Geometry check sheet. Reference: drawing and pictorial views, mm from the part's lowest x, y, z. Give positions to 0.01 mm unless a question says otherwise; leave off trailing zeros. Loops run counter-clockwise (first coordinate to the right, second up) from the corner with the lowest first, then second, coordinate; pieces in that order, holes last. Notation, with made-up numbers: (-14.75, 3.5) - (-5.75, 3.5) arc R28 ccw to (-5.75, 35.5) - close; hole circle Ø4 at (22, -36). An arc over 180 degrees is marked (long way). One line per question, with ' | ' between items. Start each with the question number.
1. Thickness scan on line 1 along Z through (x, y) = (182.5, 1.5); line 2 along X through (y, z) = (9, 563.5). Record the ranges inside material, lowest first. Write a range as from..to.
2. Section check A-A, the plane z = 652. Enter the section's corners in (x, y).
3. Section check C-C, the plane x = 187.5. Enter the section's corners in (y, z).
4. Section check B-B, the plane y = 3.5. Enter the section's corners in (x, z), then the cut area to 3 significant figures.
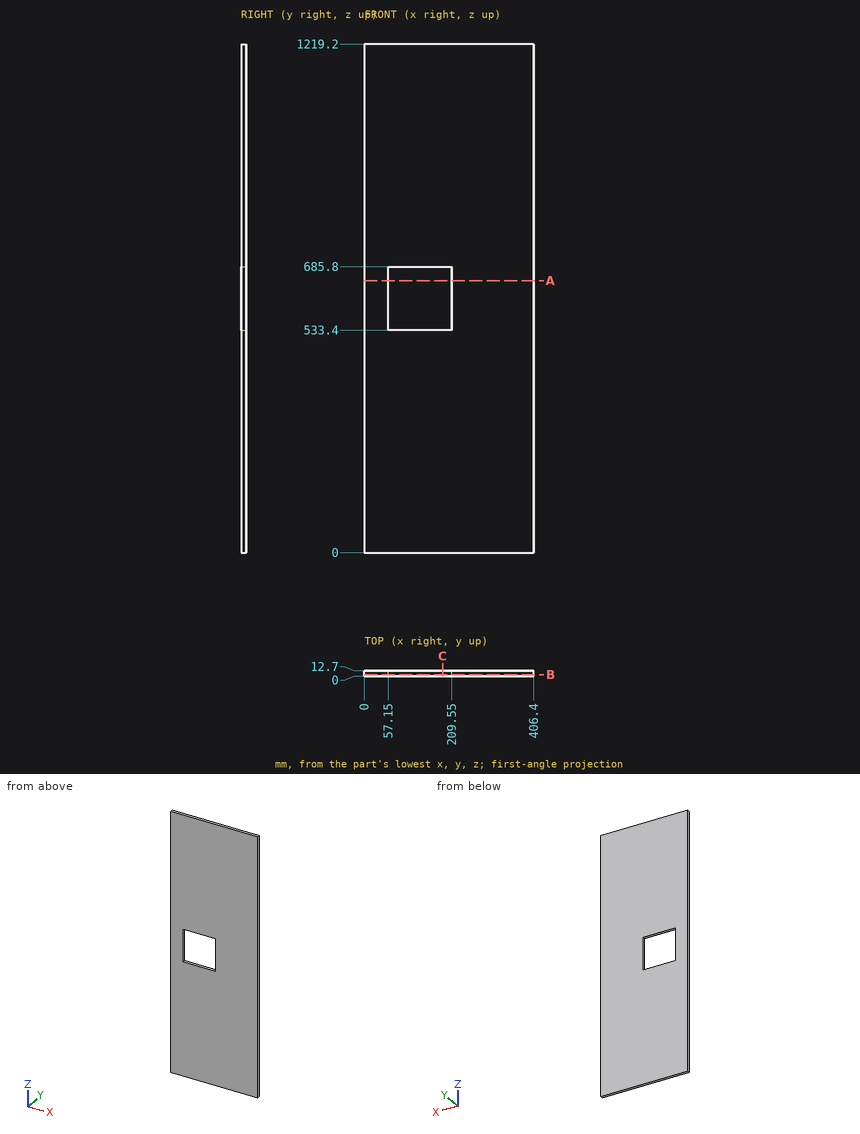
Results list:
1) line 1: 0..533.4, 685.8..1219.2 | line 2: 0..57.15, 209.55..406.4
2) outline: (0, 0) - (57.15, 0) - (57.15, 12.7) - (0, 12.7) - close; (209.55, 0) - (406.4, 0) - (406.4, 12.7) - (209.55, 12.7) - close
3) outline: (0, 0) - (12.7, 0) - (12.7, 533.4) - (0, 533.4) - close; (0, 685.8) - (12.7, 685.8) - (12.7, 1219.2) - (0, 1219.2) - close
4) outline: (0, 0) - (406.4, 0) - (406.4, 1219.2) - (0, 1219.2) - close; hole (57.15, 533.4) - (209.55, 533.4) - (209.55, 685.8) - (57.15, 685.8) - close | area: 472,000 mm²
